Can you work these out from the model? Positions are in its coordinate system, mm. A direction names the side the tool comes from. Give positions to 0.01 mm unless a question says otherwise; leave off trailing zeros. Loops run counter-clockwise (first coordinate to the right, second up) from the corner with the lowest first, then second, coordinate; pieces in that order, holes last. Notation, with made-up numbers: M -33,28 L -7,28 A13 cw -7,39 Z; hole C 20.5,25.25 d1. An arc over 180 degrees is marked long. Put each result on its own line as item: value. Start each with the question number.
1) Imagine slicing it at C-C (z = 4). Write out the boundary of the cut face in (x, y), then the cut area to 3 significant figures.
2) Imagine slicing it at A-A (z = 7.75). Write out the boundary of the cut face in (x, y), then the cut area to 3 significant figures.
3) Imagine slicing it at D-D (x = -25). Write out the boundary of the cut face in (y, z).
4) For P1, Ø3, axis at y = 0, z = 6.5, coming from the +X side; P2, Ø1.1, axis at x = -27.5, y = -4.5, coming from the +Z side; P3, Ø3, axis at y = 12, z = 3.5, coming from the -X side, each with a flat end and sliding along its axis, tell me the tip position at first contact or that it passes through.
5) For faces 1 (the flat face through (-27, -1, 5)), 2 (the flat face through (-21.694, -2, 4)), 3 (the flat face through (-15, 12, 5)), which set-ups out of +Z, -Z, +X, -X, +Y, -Y let a thin tool reach every point of the face, with its end or its side?
6) If we mould it in two halves opening along X, with no side actions, what happens to faces 4 (the flat face through (-21, 8, 0)), 5 (the flat face through (-29.23, -1, 7)), 6 (the flat face through (-5.024, 11, 3)), 7 (the flat face through (-24.074, 12, 3))? For each: +X half, -X half, draft (parallel to the pull), parting line (faces both ways), or undercut.
7) Imagine slicing it at B-B (y = -1.25). Write out the boundary of the cut face in (x, z).
8) Please list where these lines run through material, in increasing order: line 1 along X through (y, z) = (-2, 5.75); line 2 along Y through (x, z) = (-12.5, 6.5); line 3 along X through (y, z) = (7.25, 7). Write a range as from..to.
Autodesk Inventor part; units mm, degrees
ref_plane "YZ Plane" through (0, 0, 0) normal (1, 0, 0) x (0, 1, 0)
ref_plane "XZ Plane" through (0, 0, 0) normal (0, 1, 0) x (-1, 0, 0)
ref_plane "XY Plane" through (0, 0, 0) normal (0, 0, 1) x (1, 0, 0)
sketch "Sketch1" plane through (0, 0, 0) normal (0, 0, 1) x (1, 0, 0)
  line L0 (-30.4239, 15.0503) -> (-5.0239, 15.0503)
  line L1 (-5.0239, 15.0503) -> (-5.0239, -10.3497)
  line L2 (-5.0239, -10.3497) -> (-30.4239, -10.3497)
  line L3 (-30.4239, -10.3497) -> (-30.4239, 15.0503)
  point P0 (0, 0)
  dimension "d0" = 25.4
  dimension "d1" = 25.4
extrude "Extrusion1" add sketch "Sketch1" along normal blind 6.6
sketch "Sketch2" plane through (0, 0, 6.6) normal (0, 0, 1) x (1, 0, 0)
  line L0 (-5.0239, 15.0503) -> (-30.4239, 15.0503)
  line L1 (-30.4239, 15.0503) -> (-24.0739, 15.0503)
  line L2 (-24.0739, 15.0503) -> (-24.0739, 8.7003)
  line L3 (-24.0739, 8.7003) -> (-30.4239, 8.7003)
  line L4 (-30.4239, 8.7003) -> (-30.4239, 15.0503)
  point P0 (0, 0)
  dimension "d4" = 6.35
  dimension "d5" = 6.35
extrude "Extrusion2" cut sketch "Sketch2" against normal blind 6.6
sketch "Sketch3" plane through (0, 0, 6.6) normal (0, 0, 1) x (1, 0, 0)
  line L0 (-5.0239, 15.0503) -> (-24.0739, 15.0503)
  line L1 (-24.0739, 8.7003) -> (-24.0739, 15.0503) construction
  line L2 (-24.0739, 15.0503) -> (-24.0739, 8.7003) construction
  line L3 (-30.4239, 8.7003) -> (-24.0739, 8.7003) construction
  line L4 (-24.0739, 8.7003) -> (-30.4239, 8.7003) construction
  line L5 (-27.2489, 8.7003) -> (-27.2489, -10.3839) construction
  line L6 (-24.0739, 11.8753) -> (-5.0239, 11.8753) construction
  line L7 (-5.0239, -10.3497) -> (-5.0239, 15.0503)
  line L8 (-5.0239, 13.5009) -> (-5.0239, 10.2497)
  line L9 (-5.0239, 10.2497) -> (-24.0739, 10.2497)
  line L10 (-24.0739, 10.2497) -> (-24.0739, 13.5009)
  line L11 (-30.4239, -10.3497) -> (-5.0239, -10.3497)
  line L12 (-28.8745, 8.7003) -> (-25.6233, 8.7003)
  line L13 (-25.6233, 8.7003) -> (-25.6233, -10.3497)
  line L14 (-25.6233, -10.3497) -> (-28.8745, -10.3497)
  line L15 (-28.8745, -10.3497) -> (-29.2301, -10.3497)
  line L16 (-29.2301, -10.3497) -> (-29.2301, 8.7003)
  line L17 (-28.8745, 8.7003) -> (-29.2301, 8.7003)
  line L18 (-24.0739, 13.5009) -> (-24.0739, 13.8565)
  line L19 (-24.0739, 13.8565) -> (-5.0239, 13.8565)
  line L20 (-5.0239, 13.8565) -> (-5.0239, 13.5009)
  point P0 (0, 0)
  dimension "d8" = 3.2512
  dimension "d20" = 0.3556
  dimension "d21" = 0.3556
extrude "Extrusion3" cut sketch "Sketch3" against normal blind 1.6
sketch "Sketch4" plane through (0, 0, 6.6) normal (0, 0, 1) x (1, 0, 0)
  line L0 (-24.0739, 8.7003) -> (-25.6233, 8.7003)
  line L1 (-25.6233, 8.7003) -> (-24.0739, 8.7003)
  line L2 (-5.0239, 10.2497) -> (-24.0739, 10.2497)
  line L3 (-24.0739, 8.7003) -> (-24.0739, 10.2497)
  line L4 (-24.0739, 10.2497) -> (-5.0239, 10.2497)
  line L5 (-5.0239, -10.3497) -> (-5.0239, 10.2497)
  line L6 (-5.0239, 10.2497) -> (-5.0239, -10.3497)
  line L7 (-5.0239, -10.3497) -> (-25.6233, -10.3497)
  line L8 (-5.0239, -10.3497) -> (-30.4239, -10.3497)
  line L9 (-25.6233, 8.7003) -> (-25.6233, -10.3497)
  point P0 (0, 0)
extrude "Extrusion4" add sketch "Sketch4" along normal blind 2
sketch "Sketch5" plane through (0, 0, 6.6) normal (0, 0, 1) x (1, 0, 0)
  line L0 (-5.0239, 15.0503) -> (-24.0739, 15.0503)
  line L1 (-24.0739, 15.0503) -> (-5.0239, 15.0503)
  line L2 (-30.4239, -10.3497) -> (-30.4239, 8.7003)
  line L3 (-30.4239, 8.7003) -> (-29.2301, 8.7003)
  line L4 (-30.4239, 8.7003) -> (-24.0739, 8.7003)
  line L5 (-29.2301, 8.7003) -> (-29.2301, -10.3497)
  line L6 (-30.4239, -10.3497) -> (-29.2301, -10.3497)
  line L7 (-29.2301, -10.3497) -> (-30.4239, -10.3497)
  line L8 (-24.0739, 15.0503) -> (-24.0739, 13.8565)
  line L9 (-24.0739, 15.0503) -> (-24.0739, 13.8565)
  line L10 (-24.0739, 13.8565) -> (-5.0239, 13.8565)
  line L11 (-5.0239, 13.8565) -> (-5.0239, 15.0503)
  point P0 (0, 0)
  point P1 (-5.0239, 13.5009)
  point P2 (-28.8745, -10.3497)
  point P3 (-24.0739, 13.5009)
  dimension "d18" = 1.1938
  dimension "d19" = 1.1938
extrude "Extrusion5" add sketch "Sketch5" along normal blind 2
sketch "Sketch6" plane through (0, 0, 8.6) normal (0, 0, 1) x (1, 0, 0)
  line L0 (-25.6233, -10.3497) -> (-5.0239, -10.3497)
  line L1 (-5.0239, -10.3497) -> (-21.6937, -10.3497)
  line L2 (-21.6937, -10.3497) -> (-21.6937, 6.1438)
  line L3 (-21.6937, 6.1438) -> (-5.0239, 6.1438)
  line L4 (-5.0239, 6.1438) -> (-5.0239, -10.3497)
  point P0 (0, 0)
extrude "Extrusion6" cut sketch "Sketch6" against normal blind 9
properties part number "BalsaJig"
Recorded:
1. outline: M -30.42,-10.35 L -21.69,-10.35 L -21.69,6.14 L -5.02,6.14 L -5.02,15.05 L -24.07,15.05 L -24.07,8.7 L -30.42,8.7 Z
1. area: 330 mm²
2. outline: M -30.42,-10.35 L -29.23,-10.35 L -29.23,8.7 L -30.42,8.7 Z; M -25.62,-10.35 L -21.69,-10.35 L -21.69,6.14 L -5.02,6.14 L -5.02,10.25 L -24.07,10.25 L -24.07,8.7 L -25.62,8.7 Z; M -24.07,13.86 L -5.02,13.86 L -5.02,15.05 L -24.07,15.05 Z
2. area: 192 mm²
3. outline: M -10.35,0 L 8.7,0 L 8.7,8.6 L -10.35,8.6 Z
4. P1: x = -21.69
4. P2: z = 5
4. P3: x = -24.07
5. face 1: +Z, +Y, -Y
5. face 2: +Z, -Z, +X, -Y
5. face 3: +Z, +X, -X
6. face 4: draft
6. face 5: undercut
6. face 6: +X half
6. face 7: -X half
7. outline: M -30.42,0 L -21.69,0 L -21.69,8.6 L -25.62,8.6 L -25.62,5 L -29.23,5 L -29.23,8.6 L -30.42,8.6 Z
8. line 1: -30.42..-29.23, -25.62..-21.69
8. line 2: 6.14..10.25, 13.86..15.05
8. line 3: -30.42..-29.23, -25.62..-5.02
